Job drawing, mm, ordinate dimensions from the low corner. One solid piece. A direction names the side the tool comes from. Give positions to 0.01 mm unless a question says otherwise; leave off trailing zeros. Loops run counter-clockwise (first coordinate to the right, second up) from the corner with the lowest first, then second, coordinate; pieces in that order, holes last. Notation, with made-up numbers: (36, 86) -> (80, 86) arc R27 ccw to (80, 114) -> close; hole circle Ø2 at (70, 58.25). An arc over 180 degrees is marked (long way). Use one line per item in the form item = value.
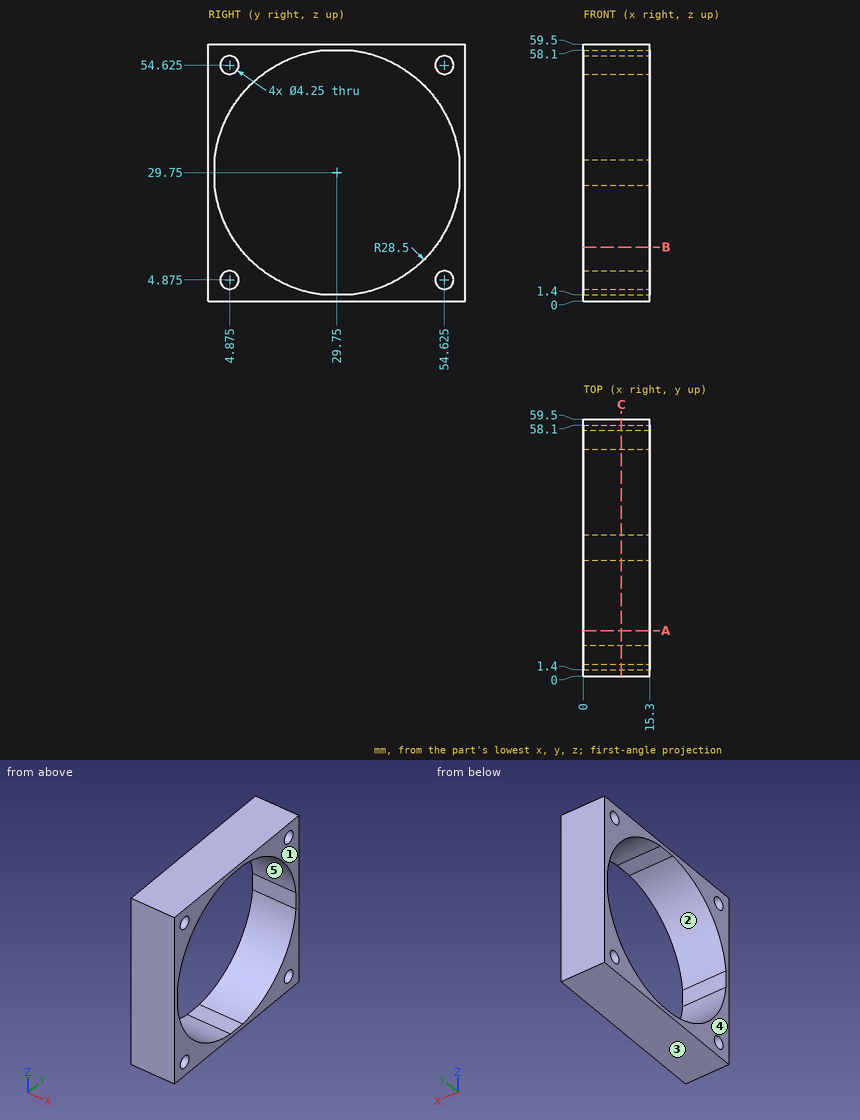
1. Tool access for the marked faces 4 and 5: list every direction of +Z, -Z, +X, -X, +Y, -Y with a clear straight run to the whole face (end or side of a thin tool).
Result sheet:
face_4 = +Z, -Z, -X, +Y, -Y
face_5 = +X, -X
2. Mould opens along Z. For the marked faces 1, 2 and 3 say: pulls with the +Z half, pulls with the -Z half, needs draft (parallel to the pull), parting line crosses it, or undercut.
Result sheet:
face_1 = needs draft
face_2 = undercut
face_3 = pulls with the -Z half
3. Cut at C-C, the plane x = 8.75. Write the cut outline in (y, z) (3 decimals).
Result sheet:
outline = (0, 0) -> (59.5, 0) -> (59.5, 59.5) -> (0, 59.5) -> close; hole (1.4, 26.83) arc R28.5 ccw to (26.83, 1.4) -> (32.67, 1.4) arc R28.5 ccw to (58.1, 26.83) -> (58.1, 32.67) arc R28.5 ccw to (32.67, 58.1) -> (26.83, 58.1) arc R28.5 ccw to (1.4, 32.67) -> close; hole circle Ø4.25 at (4.875, 4.875); hole circle Ø4.25 at (4.875, 54.625); hole circle Ø4.25 at (54.625, 4.875); hole circle Ø4.25 at (54.625, 54.625)
4. Cut at B-B, the plane z = 12.5. Write the cut outline in (x, y), then the cut area to 3 significant figures.
Result sheet:
outline = (0, 0) -> (15.3, 0) -> (15.3, 7.06) -> (0, 7.06) -> close; (0, 52.44) -> (15.3, 52.44) -> (15.3, 59.5) -> (0, 59.5) -> close
area = 216 mm^2
5. Drill centre lines: line 1 (Z direction, x = 2.5, y = 30); line 2 (Z direction, x = 1, y = 5); line 3 (Z direction, x = 4.25, y = 5.5). Where is each one in solid material? Low to high.
Result sheet:
line_1 = 0 to 1.4, 58.1 to 59.5
line_2 = 0 to 2.75, 7 to 15.62, 43.88 to 52.5, 56.75 to 59.5
line_3 = 0 to 2.84, 6.91 to 14.78, 44.72 to 52.59, 56.66 to 59.5
6. Cut at A-A, the plane y = 10.5. Write the cut outline in (x, z), then the cut area to 3 significant figures.
Result sheet:
outline = (0, 0) -> (15.3, 0) -> (15.3, 8.73) -> (0, 8.73) -> close; (0, 50.77) -> (15.3, 50.77) -> (15.3, 59.5) -> (0, 59.5) -> close
area = 267 mm^2
